```python
from build123d import *

# Parameters (mm, degrees)
F0_W      = 14
F0_H      = 36
F1_DEPTH  = 12
F2_R      = 7.5
F3_DEPTH  = 36.001
F5_W      = 28
F5_H      = 8
F6_DEPTH  = 11
F7_R      = 3
F8_R      = 5
F9_SIZE   = 1
F10_R     = 1
F11_DEPTH = 4
F12_R     = 1
F13_DEPTH = 5


with BuildPart() as f1:
    # F0 (on Top) → F1 (new body)
    with BuildSketch(Plane.XY):
        Rectangle(F0_W, F0_H)
    extrude(amount=F1_DEPTH)

    # F2 (on face) → F3 (cut, through all)
    with BuildSketch(Plane.XZ.offset(18)):
        with Locations((-12.5, 6)):
            Circle(F2_R)
    extrude(amount=-F3_DEPTH, mode=Mode.SUBTRACT)

    # F5 (on offset) → F6 (cut)
    with BuildSketch(Plane.YZ.offset(-7)):
        with Locations((0, 6)):
            Rectangle(F5_W, F5_H)
    extrude(amount=F6_DEPTH, mode=Mode.SUBTRACT)

    # F7
    f7_edges = [f1.edges().sort_by_distance(p)[0] for p in [
        (-1.077856, 14, 2),
        (-1.077856, -14, 10),
        (-1.077856, -14, 2),
        (-1.077856, 14, 10),
    ]]
    fillet(f7_edges, radius=F7_R)

    # F8
    f8_edges = [f1.edges().sort_by_distance(p)[0] for p in [
        (7, -18, 6),
        (7, 18, 6),
    ]]
    fillet(f8_edges, radius=F8_R)

    # F9
    f9_edges = [f1.edges().sort_by_distance(p)[0] for p in [
        (-2.5, -18, 0),
        (-2.5, -18, 12),
    ]]
    chamfer(f9_edges, length=F9_SIZE)

    # F10 (on face) → F11 (cut, through all)
    with BuildSketch(Plane(origin=(0, 18, 0), x_dir=(-1, 0, 0), z_dir=(0, 1, 0))):
        with Locations((0, 6)):
            Circle(F10_R)
    extrude(amount=-F11_DEPTH, mode=Mode.SUBTRACT)

    # F12 (on offset) → F13 (cut)
    with BuildSketch(Plane.YZ.offset(-7)):
        with Locations((-16, 4)):
            Circle(F12_R)
        with Locations((16, 2)):
            Circle(F12_R)
    extrude(amount=F13_DEPTH, mode=Mode.SUBTRACT)


solid = f1.part
```
Read the model definition and answer for the solid it produces. Units are mm, in the model's axes. A direction names the side the tool comes from. Give positions to 0.01 mm unless a question says otherwise; leave off trailing zeros. Write each loop counter-clockwise with the first axis right and the second up, starting at its lowest first coordinate (ties: lowest second). Pieces come first, ordered by that corner, then holes. Notation, with made-up numbers: (-23.75, 58.25) -> (-11.75, 58.25) arc R13 cw to (-11.75, 66.25) -> close; hole circle Ø3 at (25.5, 25.5). An arc over 180 degrees is marked (long way). Answer as a JSON object with one key per item and string values.
1) Straight lines are drawn through the part: probe 1 along Z at (x, y) = (-2.85, -16); probe 2 along Z at (x, y) = (3.5, 3); probe 3 along Y at (x, z) = (-3.25, 4.5). For each, find the intervals that lie inside material, in ascending order. Write a range as from..to.
Findings below:
{"probe 1": "z = 0..3, 5..12", "probe 2": "z = 0..2, 10..12", "probe 3": "y = -18..-16.87, -15.13..-13.96, 13.96..18"}
2) Section C-C on y = 5.5 is taken. Write down the section's boundary in (x, z).
Findings below:
{"outline": "(-7, 0) -> (6, 0) -> (7, 1) -> (7, 11) -> (6, 12) -> (-7, 12) -> (-7, 11.1) arc R7.5 cw to (-6.16, 10) -> (4, 10) -> (4, 2) -> (-6.16, 2) arc R7.5 cw to (-7, 0.9) -> close"}
3) A tool of negligible diameter and unlimited length cuts with its end or side. For faces 4 (the flat face through (4, 0, 6)), 5 (the flat face through (-2, -18, 6)), from which of +Z, -Z, +X, -X, +Y, -Y can it reach the whole face along a straight path? Write none if from no direction.
Findings below:
{"face 4": "-X", "face 5": "+Z, -Z, +X, -X, -Y"}
4) Section B-B on x = -2.5 is taken. Write down the section's boundary in (y, z), then the cut area to 3 significant figures.
Findings below:
{"outline": "(-18, 1) -> (-17, 0) -> (17, 0) -> (18, 1) -> (18, 11) -> (17, 12) -> (-17, 12) -> (-18, 11) -> close; hole circle Ø2 at (-16, 4); hole (-14, 5) arc R3 ccw to (-11, 2) -> (11, 2) arc R3 ccw to (14, 5) -> (14, 7) arc R3 ccw to (11, 10) -> (-11, 10) arc R3 ccw to (-14, 7) -> close; hole circle Ø2 at (16, 2)", "area": "207 mm^2"}
5) Flat-ended cylindrical pins translate along their axes: pin 1 Ø1.5 at (y, z) = (13, 3) entering from -X; pin 2 Ø2 at (y, z) = (-16, 4.5) entering from -X; pin 3 Ø4 at (y, z) = (2, 5.5) entering from -X; pin 4 Ø6 at (x, z) = (-5.5, 6.5) entering from +Y. Find the tip coordinate at first contact, or state that the pin passes through.
Findings below:
{"pin 1": "stops at x = -6", "pin 2": "stops at x = -5.21", "pin 3": "stops at x = 4", "pin 4": "stops at y = 18"}
6) Section D-D on z = 1.5 is taken. Write down the section's boundary in (x, y), then the cut area to 3 significant figures.
Findings below:
{"outline": "(-6.5, -18) -> (2, -18) arc R5 ccw to (7, -13) -> (7, 13) arc R5 ccw to (2, 18) -> (-6.5, 18) -> (-6.5, 16.87) -> (-2, 16.87) -> (-2, 15.13) -> (-6.5, 15.13) -> close", "area": "467 mm^2"}
7) Section A-A on z = 6 is taken. Write down the section's boundary in (x, y).
Findings below:
{"outline": "(-5, -18) -> (2, -18) arc R5 ccw to (7, -13) -> (7, 13) arc R5 ccw to (2, 18) -> (1, 18) -> (1, 14) -> (4, 14) -> (4, -14) -> (-5, -14) -> close; (-5, 14) -> (-1, 14) -> (-1, 18) -> (-5, 18) -> close"}
8) For a pull along Y with two mould halves and no side action, classify faces 1 (the flat face through (-2.4, 17.5, 11.5)), 2 (the flat face through (6.5, -0.2, 11.5)), 3 (the cylindrical face through (-4, 16, 1)) as pulls with the +Y half, pulls with the -Y half, needs draft (parallel to the pull), parting line crosses it, or undercut.
Findings below:
{"face 1": "pulls with the +Y half", "face 2": "needs draft", "face 3": "undercut"}
